The model under review builds one solid part; all positions refer to its coordinate system, in mm. A direction names the side the tool comes from. Coordinates: 2 decimals unless noted, no trailing zeros. Order: outer loops, then holes, each group sorted by start corner. A loop starts at its lowest first (then second) coordinate and runs counter-clockwise, first axis right, second up. Notation, with made-up numbers: (73.25, -19.5) -> (81.25, -19.5) arc R18 ccw to (81.25, -10.5) -> close; hole circle Ø1 at (76.25, 9.25). An arc over 180 degrees is marked (long way). Put each result on its own line as item: value.
from build123d import *

# Parameters (mm, degrees)
ESQUISSE1_R        = 1.4
BOSS_EXTRU_1_DEPTH = 2.1
ESQUISSE2_R        = 0.8
BOSS_EXTRU_2_DEPTH = 5.6
ESQUISSE3_R        = 1.4
BOSS_EXTRU_3_DEPTH = 2.1
BOSS_EXTRU_4_START = -2.3
ESQUISSE4_R        = 1.25
BOSS_EXTRU_4_DEPTH = 1


with BuildPart() as part:
    # Esquisse1 → Boss.-Extru.1 (new body)
    with BuildSketch(Plane.XY):
        with Locations((4, 14.075)):
            Circle(ESQUISSE1_R)
    extrude(amount=BOSS_EXTRU_1_DEPTH)

    # Esquisse2 → Boss.-Extru.2 (add)
    with BuildSketch(Plane.XY.offset(2.1)):
        with Locations((4, 14.075)):
            Circle(ESQUISSE2_R)
    extrude(amount=BOSS_EXTRU_2_DEPTH)

    # Esquisse3 → Boss.-Extru.3 (add)
    with BuildSketch(Plane.XY.offset(7.7)):
        with Locations((4, 14.075)):
            Circle(ESQUISSE3_R)
    extrude(amount=BOSS_EXTRU_3_DEPTH)

    # Esquisse4 → Boss.-Extru.4 (add)
    with BuildSketch(Plane(origin=(0, 0, 0), x_dir=(-1, 0, 0), z_dir=(0, 0, -1)).offset(BOSS_EXTRU_4_START)):
        with Locations((-4, 14.075)):
            Circle(ESQUISSE4_R)
    extrude(amount=-BOSS_EXTRU_4_DEPTH)


solid = part.part
Item 1: Consider section B-B on x = 4.9. Write out the cut boundary in (y, z).
Answers below:
outline: (13, 0) -> (15.15, 0) -> (15.15, 2.1) -> (13, 2.1) -> close; (13, 7.7) -> (15.15, 7.7) -> (15.15, 9.8) -> (13, 9.8) -> close; (13.21, 2.3) -> (14.94, 2.3) -> (14.94, 3.3) -> (13.21, 3.3) -> close
Item 2: For line 1 (Z direction, x = 3.5, y = 13.3); line 2 (Y direction, x = 3.95, z = 2.25); line 3 (X direction, y = 13.7, z = 1.25), list the stretches that pass through material, from the lowest coordinate up. Write a range as from..to.
Answers below:
line 1: 0..2.1, 2.3..3.3, 7.7..9.8
line 2: 13.28..14.87
line 3: 2.65..5.35
Item 3: Mouldability with a two-part tool opening along Z and no side actions: class faces 1 (the cylindrical face through (3.697, 12.708, 8.735)), 2 (the cylindrical face through (3.8, 13.3, 5.5)), 3 (the flat face through (4, 14, 9.8)) as +Z half, -Z half, draft (parallel to the pull), parting line (faces both ways), or undercut.
Answers below:
face 1: draft
face 2: undercut
face 3: +Z half
Item 4: For pin 1 Ø1.5 at (y, z) = (13, 4.5) entering from +X; pin 2 Ø1.5 at (y, z) = (13, 8) entering from -X, all flat-tipped, find the tip position at first contact; note any pin that passes through.
Answers below:
pin 1: x = 4.73
pin 2: x = 2.64
Item 5: Consider section D-D on z = 1.5. Write out the cut boundary in (x, y) (3 decimals).
Answers below:
outline: circle Ø2.8 at (4, 14.075)
Item 6: Consider section A-A on x = 4. Write out the cut boundary in (y, z) (3 decimals).
Answers below:
outline: (12.675, 0) -> (15.475, 0) -> (15.475, 2.1) -> (14.875, 2.1) -> (14.875, 2.3) -> (15.325, 2.3) -> (15.325, 3.3) -> (14.875, 3.3) -> (14.875, 7.7) -> (15.475, 7.7) -> (15.475, 9.8) -> (12.675, 9.8) -> (12.675, 7.7) -> (13.275, 7.7) -> (13.275, 3.3) -> (12.825, 3.3) -> (12.825, 2.3) -> (13.275, 2.3) -> (13.275, 2.1) -> (12.675, 2.1) -> close
Item 7: For faces 4 (the flat face through (4, 14, 0)), 5 (the cylindrical face through (4.163, 15.314, 2.793)), list the 3-axis set-ups (+Z, -Z, +X, -X, +Y, -Y) from which the entire face can be reached by the end or side of a thin tool; tool diameter is ignored.
Answers below:
face 4: -Z, +X, -X, +Y, -Y
face 5: none
Item 8: Consider section C-C on y = 14.55. Write out the cut boundary in (x, z).
Answers below:
outline: (2.68, 0) -> (5.32, 0) -> (5.32, 2.1) -> (4.64, 2.1) -> (4.64, 2.3) -> (5.16, 2.3) -> (5.16, 3.3) -> (4.64, 3.3) -> (4.64, 7.7) -> (5.32, 7.7) -> (5.32, 9.8) -> (2.68, 9.8) -> (2.68, 7.7) -> (3.36, 7.7) -> (3.36, 3.3) -> (2.84, 3.3) -> (2.84, 2.3) -> (3.36, 2.3) -> (3.36, 2.1) -> (2.68, 2.1) -> close
